The model under review builds one solid part; all positions refer to its coordinate system, in mm. A direction names the side the tool comes from. Coordinates: 2 decimals unless noted, no trailing zeros. Loops run counter-clockwise (first coordinate to the right, second up) from the corner with the lowest first, then second, coordinate; pieces in that order, holes last. Notation, with made-up numbers: (-36.75, -23) - (-13.75, -23) arc R31 ccw to (-13.75, 13) - close; hole circle Ø9 at (4, -14.5). An arc over 180 degrees is marked (long way). One line per item, written item: value. Start each with the question number.
1. We need section A-A, the plane z = -35. Give the boundary of the cut face in (x, y).
2. For faces 4 (the face through (3.131, -25.823, -16.71)), 5 (the face through (3, -26, 35)), list the 3-axis set-ups (+Z, -Z, +X, -X, +Y, -Y) from which the entire face can be reached by the end or side of a thin tool; tool diameter is ignored.
3. We need section C-C, the plane x = 2.25. Count the separate pieces of the cut face and the enclosed holes in it, then the cut area to 3 significant figures.
4. Insertion check: P1, Ø2.5, axis at y = -9.224, z = -45.205, coming from the +X side. The pin has a flat end and moves straight along its axis. Give the tip position at first contact, or say it passes through.
5. We need section D-D, the plane z = -10. Give the boundary of the cut face in (x, y).
6. Mouldability with a two-part tool opening along Y and no side actions: class faces 1 (the face through (3.22, -10.18, -45.81)), 2 (the face through (3, -21, 0)), 3 (the face through (3, 42.97, 0)) as +Y half, -Y half, draft (parallel to the pull), parting line (faces both ways), or undercut.
7. We need section B-B, the plane z = 22. Give the boundary of the cut face in (x, y).
8. To check wall thickness, follow line 1 (Y direction, x = 1.5, z = -49); line 2 (Y direction, x = 4.25, z = 22); line 3 (Z direction, x = 3.5, y = 13). State the ranges of each line that lie inside material, in increasing order.
from build123d import *

# Parameters (mm, degrees)
SKETCH1_W                 = 112
SKETCH1_H                 = 77
BOSS_EXTRUDE1_DEPTH       = 6.35
F_6_CLEARANCE_HOLE1_D     = 3.6576
SKETCH5_R                 = 5
CUT_EXTRUDE1_DEPTH        = 7.35
F_6_CLEARANCE_HOLE2_D     = 3.6576
F_10_CLEARANCE_HOLE1_D    = 4.9784
F_8_CLEARANCE_HOLE2_D     = 4.3053
CUT_EXTRUDE2_DEPTH        = 7.35
F_6_CLEARANCE_HOLE3_D     = 3.6576
FILLET2_R                 = 2
SKETCH25_R                = 30
CUT_EXTRUDE3_DEPTH        = 7.35
FILLET1_R                 = 5
TAP_DRILL_FOR_4_40_TAP1_D = 2.2606


with BuildPart() as part:
    # Sketch1 → Boss-Extrude1 (new body)
    with BuildSketch(Plane(origin=(0, 0, 0), x_dir=(0, 0, -1), z_dir=(1, 0, 0))):
        with Locations((0, 12.5)):
            Rectangle(SKETCH1_W, SKETCH1_H)
    extrude(amount=BOSS_EXTRUDE1_DEPTH)

    # #6 Clearance Hole1 (through all)
    with Locations(Plane(origin=(6.35, 0, 0), x_dir=(0, 0, -1), z_dir=(1, 0, 0))):
        with Locations((-22, 22), (22, 22), (22, -22), (-22, -22)):
            Hole(F_6_CLEARANCE_HOLE1_D / 2)

    # Sketch5 → Cut-Extrude1 (cut, through all)
    with BuildSketch(Plane(origin=(6.35, 0, 0), x_dir=(0, 0, -1), z_dir=(1, 0, 0))):
        Circle(SKETCH5_R)
    extrude(amount=-CUT_EXTRUDE1_DEPTH, mode=Mode.SUBTRACT)

    # #6 Clearance Hole2 (through all)
    with Locations(Plane(origin=(6.35, 0, 0), x_dir=(0, 0, -1), z_dir=(1, 0, 0))):
        with Locations((-41.914797213, 11.914797213), (-28.085202787, 11.914797213), (-28.085202787, -1.914797213), (-41.914797213, -1.914797213), (28.085202787, 11.914797213), (28.085202787, -1.914797213), (41.914797213, -1.914797213), (41.914797213, 11.914797213), (-35, 5), (35, 5)):
            Hole(F_6_CLEARANCE_HOLE2_D / 2)

    # #10 Clearance Hole1 (through all)
    with Locations(Plane.ZY):
        with Locations((18.25, 0), (-18.25, 0)):
            Hole(F_10_CLEARANCE_HOLE1_D / 2)

    # #8 Clearance Hole2 (through all)
    with Locations(Plane(origin=(0, 45.97, 49), x_dir=(0, 0, -1), z_dir=(-1, 0, 0))):
        with Locations((0, 0), (18, 0), (18, 24), (0, 24), (80, 0), (80, 24), (98, 24), (98, 0)):
            Hole(F_8_CLEARANCE_HOLE2_D / 2)

    # Sketch22 → Cut-Extrude2 (cut, through all)
    with BuildSketch(Plane.ZY):
        Polygon((12.7, 51), (-12.7, 51), (-12.6, 42.97), (12.6, 42.97), align=None)
    extrude(amount=-CUT_EXTRUDE2_DEPTH, mode=Mode.SUBTRACT)

    # #6 Clearance Hole3 (through all)
    with Locations(Plane(origin=(0, 32.5052, 10), x_dir=(0, 0, -1), z_dir=(-1, 0, 0))):
        with Locations((0, 0), (20, 0)):
            Hole(F_6_CLEARANCE_HOLE3_D / 2)

    # Fillet2
    fillet2_edges = [part.edges().sort_by_distance(p)[0] for p in [
        (3.175, 51, 12.7),
        (3.175, 51, -12.7),
    ]]
    fillet(fillet2_edges, radius=FILLET2_R)

    # Sketch25 → Cut-Extrude3 (cut, through all)
    with BuildSketch(Plane.ZY):
        with Locations((0, -51)):
            Circle(SKETCH25_R)
    extrude(amount=-CUT_EXTRUDE3_DEPTH, mode=Mode.SUBTRACT)

    # Fillet1
    fillet1_edges = [part.edges().sort_by_distance(p)[0] for p in [
        (3.175, -26, -16.583123952),
        (3.175, -26, 16.583123952),
        (3.175, -26, -56),
        (3.175, -26, 56),
    ]]
    fillet(fillet1_edges, radius=FILLET1_R)

    # Tap Drill for #4-40 Tap1 (through all)
    with Locations(Plane(origin=(0, -21.924, 45.205), x_dir=(0, 0, -1), z_dir=(-1, 0, 0))):
        with Locations((0, 0), (0, -12.7)):
            tap_drill_for_4_40_tap1 = Hole(TAP_DRILL_FOR_4_40_TAP1_D / 2)

    # Mirror1: Tap Drill for #4-40 Tap1 across plane
    add(tap_drill_for_4_40_tap1.mirror(Plane.XY), mode=Mode.SUBTRACT)


solid = part.part
Findings below:
1. outline: (0, -26) - (6.35, -26) - (6.35, 3.17) - (0, 3.17) - close; (0, 6.83) - (6.35, 6.83) - (6.35, 51) - (0, 51) - close
2. face 4: +X, -X, -Y
2. face 5: +Z, -Z, +X, -X, -Y
3. separate pieces: 1
3. enclosed holes: 31
3. area: 7,880 mm2
4. P1: x = 6.35
5. outline: (0, -22.72) - (6.35, -22.72) - (6.35, 30.68) - (0, 30.68) - close; (0, 34.33) - (6.35, 34.33) - (6.35, 42.97) - (0, 42.97) - close
6. face 1: undercut
6. face 2: -Y half
6. face 3: +Y half
7. outline: (0, -26) - (6.35, -26) - (6.35, -23.83) - (0, -23.83) - close; (0, -20.17) - (6.35, -20.17) - (6.35, 20.17) - (0, 20.17) - close; (0, 23.83) - (6.35, 23.83) - (6.35, 51) - (0, 51) - close
8. line 1: -26 to 19.82, 24.12 to 43.82, 48.12 to 51
8. line 2: -26 to -23.83, -20.17 to 20.17, 23.83 to 51
8. line 3: -56 to -43.39, -40.44 to -29.56, -26.61 to 26.61, 29.56 to 40.44, 43.39 to 56
